Design review of the part built by this model. Coordinates are the model's own, in mm. Coordinates: 2 decimals unless noted, no trailing zeros. Write each loop counter-clockwise with the first axis right and the second up, starting at its lowest first coordinate (ties: lowest second). Pieces come first, ordered by that corner, then holes. Notation, with made-up numbers: (-18, 49) -> (27, 49) arc R32 cw to (27, 85) -> close; hole circle Ø5 at (-21.5, 18.5). An arc over 180 degrees is marked (long way). One line per question, with ' | ' between items. Start each with the question number.
Q1. Add section B-B on x = 57. State the section outline as (y, z) points.
Q2. Add section C-C on z = -11. State the section outline as (x, y) points, and give its area (3 significant figures).
Q3. Wall thickness on probe 1 along X at (y, z) = (-5, -90); probe 2 along X at (y, z) = (-5.5, -90.5); probe 3 along Z at (x, y) = (91, -5.5): over which ranges is each line inside the solid? List them lowest first.
Q4. Add section D-D on y = -2.5. Give the number of separate pieces and of enclosed holes in the cut face, and give its area (3 significant figures).
Q5. Add section A-A on z = -79. State the section outline as (x, y) points.
Q6. Draft analysis for pull direction Z (two halves, no side actions). For faces 1 (the flat face through (19.525, -3.131, -110.119)), 2 (the flat face through (42, 0, -54)), 3 (the cylindrical face through (61.79, -3.13, -46.69)), state which applies: pulls with the +Z half, pulls with the -Z half, needs draft (parallel to the pull), parting line crosses it, or undercut.
Q7. For P1, Ø1.5, axis at y = -1, z = -44, coming from the +X side; P2, Ø1, axis at y = -1.5, z = -109.5, coming from the +X side, all flat-tipped, find the tip position at first contact; note any pin that passes through.
from build123d import *

# Parameters (mm, degrees)
BASE_FLANGE1_DEPTH = 6.35
SKETCH8_R          = 3.4
CUT_EXTRUDE1_DEPTH = 175.95180765
SKETCH9_R          = 34
CUT_EXTRUDE2_DEPTH = 175.95180765
SKETCH10_R         = 2.5
CUT_EXTRUDE3_DEPTH = 175.95180765


# Sheet-metal steps are written as plain solids
with BuildPart() as part:
    # Sketch2 → Base-Flange1 (new body)
    with BuildSketch(Plane(origin=(0, 0, 0), x_dir=(1, 0, 0), z_dir=(0, 1, 0))):
        with BuildLine():
            Line((0, 0), (38.51093065, 0))
            Line((38.51093065, 0), (95.630465325, 57.119534675))
            ThreePointArc((95.630465325, 57.119534675), (99.287953618, 118.761570635), (38.51093065, 129.682710556))
            Line((38.51093065, 129.682710556), (0, 90))
            Line((0, 90), (0, 0))
        make_face()
    extrude(amount=-BASE_FLANGE1_DEPTH)

    # Sketch8 → Cut-Extrude1 (cut, through all)
    with BuildSketch(Plane(origin=(0, 0, 0), x_dir=(1, 0, 0), z_dir=(0, 1, 0))):
        with Locations(Location((12.5, 79, 0), (0, 0, 270))):
            Circle(SKETCH8_R)
        with Locations(Location((12.5, 11, 0), (0, 0, 90))):
            Circle(SKETCH8_R)
    extrude(amount=-CUT_EXTRUDE1_DEPTH, mode=Mode.SUBTRACT)

    # Sketch9 → Cut-Extrude2 (cut, through all)
    with BuildSketch(Plane(origin=(0, 0, 0), x_dir=(1, 0, 0), z_dir=(0, 1, 0))):
        with Locations(Location((62.75, 90, 0), (0, 0, 270))):
            Circle(SKETCH9_R)
    extrude(amount=-CUT_EXTRUDE2_DEPTH, mode=Mode.SUBTRACT)

    # Sketch10 → Cut-Extrude3 (cut, through all)
    with BuildSketch(Plane(origin=(0, 0, 0), x_dir=(1, 0, 0), z_dir=(0, 1, 0))):
        with Locations(Location((62.75, 131, 0), (0, 0, 270))):
            Circle(SKETCH10_R)
        with Locations(Location((91.741378029, 118.991378029, 0), (0, 0, 270))):
            Circle(SKETCH10_R)
        with Locations(Location((103.75, 90, 0), (0, 0, 270))):
            Circle(SKETCH10_R)
        with Locations(Location((91.741378029, 61.008621971, 0), (0, 0, 270))):
            Circle(SKETCH10_R)
        with Locations(Location((62.75, 49, 0), (0, 0, 270))):
            Circle(SKETCH10_R)
        with Locations(Location((33.758621971, 61.008621971, 0), (0, 0, 270))):
            Circle(SKETCH10_R)
        with Locations(Location((21.75, 90, 0), (0, 0, 270))):
            Circle(SKETCH10_R)
        with Locations(Location((33.758621971, 118.991378029, 0), (0, 0, 270))):
            Circle(SKETCH10_R)
    extrude(amount=-CUT_EXTRUDE3_DEPTH, mode=Mode.SUBTRACT)


solid = part.part
Output values:
1) outline: (-6.35, -136.14) -> (0, -136.14) -> (0, -123.51) -> (-6.35, -123.51) -> close; (-6.35, -56.49) -> (0, -56.49) -> (0, -18.49) -> (-6.35, -18.49) -> close
2) outline: (0, -6.35) -> (9.1, -6.35) -> (9.1, 0) -> (0, 0) -> close; (15.9, -6.35) -> (49.51, -6.35) -> (49.51, 0) -> (15.9, 0) -> close | area: 271 mm2
3) probe 1: x = 0 to 19.25, 24.25 to 28.75, 96.75 to 101.25, 106.25 to 109.25 | probe 2: x = 0.49 to 19.3, 24.2 to 28.75, 96.75 to 101.3, 106.2 to 109.25 | probe 3: z = -126.93 to -121.38, -116.6 to -108.92, -71.08 to -63.4, -58.62 to -52.49
4) separate pieces: 1 | enclosed holes: 11 | area: 6,960 mm2
5) outline: (0, -6.35) -> (9.1, -6.35) -> (9.1, 0) -> (0, 0) -> close; (15.9, -6.35) -> (30.58, -6.35) -> (30.58, 0) -> (15.9, 0) -> close; (94.92, -6.35) -> (107.93, -6.35) -> (107.93, 0) -> (94.92, 0) -> close
6) face 1: pulls with the -Z half | face 2: needs draft | face 3: undercut
7) P1: stops at x = 83.26 | P2: stops at x = 105.19
